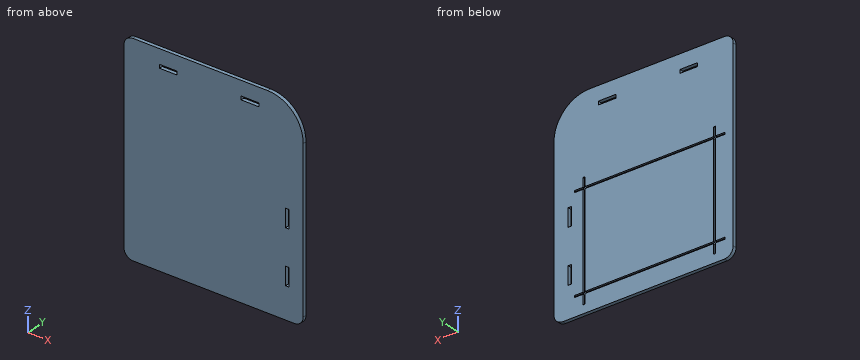
```python
from build123d import *

# Parameters (mm, degrees)
SKETCH1_W           = 20
SKETCH1_H           = 4
SKETCH1_W_2         = 4
SKETCH1_H_2         = 20
BOSS_EXTRUDE1_DEPTH = 4
SKETCH2_W           = 145
SKETCH2_H           = 105
CUT_EXTRUDE1_DEPTH  = 2


with BuildPart() as part:
    # Sketch1 → Boss-Extrude1 (new body)
    with BuildSketch(Plane(origin=(0, 0, 0), x_dir=(1, 0, 0), z_dir=(0, 1, 0))):
        with BuildLine():
            Line((-12.1, 127.1), (170, 127.1))
            ThreePointArc((170, 127.1), (177.071067812, 124.171067812), (180, 117.1))
            Line((180, 117.1), (180, -60))
            ThreePointArc((180, -60), (168.284271247, -88.284271247), (140, -100))
            Line((140, -100), (-12.1, -100))
            ThreePointArc((-12.1, -100), (-19.171067812, -97.071067812), (-22.1, -90))
            Line((-22.1, -90), (-22.1, 117.1))
            ThreePointArc((-22.1, 117.1), (-19.171067812, 124.171067812), (-12.1, 127.1))
        make_face()
        with Locations((27.9, -82)):
            Rectangle(SKETCH1_W, SKETCH1_H, mode=Mode.SUBTRACT)
        with Locations((120, -82)):
            Rectangle(SKETCH1_W, SKETCH1_H, mode=Mode.SUBTRACT)
        with Locations((162, 82.1)):
            Rectangle(SKETCH1_W_2, SKETCH1_H_2, mode=Mode.SUBTRACT)
        with Locations((162, 22.9)):
            Rectangle(SKETCH1_W_2, SKETCH1_H_2, mode=Mode.SUBTRACT)
    extrude(amount=BOSS_EXTRUDE1_DEPTH)

    # Sketch2 → Cut-Extrude1 (cut)
    with BuildSketch(Plane(origin=(0, 4, 0), x_dir=(1, 0, 0), z_dir=(0, 1, 0))):
        Polygon((-12.9, 0), (-2.1, 0), (-2.1, 105), (-12.9, 105), (-12.9, 107.1), (-2.1, 107.1), (-2.1, 117.9), (0, 117.9), (0, 107.1), (145, 107.1), (145, 117.9), (147.1, 117.9), (147.1, 107.1), (157.1, 107.1), (157.1, 105), (147.1, 105), (147.1, 0), (157.1, 0), (157.1, -2.1), (147.1, -2.1), (147.1, -12.1), (145, -12.1), (145, -2.1), (0, -2.1), (0, -12.1), (-2.1, -12.1), (-2.1, -2.1), (-12.9, -2.1), align=None)
        with Locations((72.5, 52.5)):
            Rectangle(SKETCH2_W, SKETCH2_H, mode=Mode.SUBTRACT)
    extrude(amount=-CUT_EXTRUDE1_DEPTH, mode=Mode.SUBTRACT)


solid = part.part
```
Design review of the part built by this model. Coordinates are the model's own, in mm. Round coordinates to 2 decimals unless told otherwise and drop trailing zeros. Order: outer loops, then holes, each group sorted by start corner. A loop starts at its lowest first (then second) coordinate and runs counter-clockwise, first axis right, second up. Notation, with made-up numbers: (0, -25) - (25, -25) arc R22 ccw to (25, 13) - close; hole circle Ø5 at (86.25, 81). An arc over 180 degrees is marked (long way). Return JSON: item names as keys, results as strings.
Q1. Wall thickness on L1, parallel to Z at x = 62, y = 2.05; L2, parallel to X at y = 2.1, z = 9.5; L3, parallel to Z at x = 117, y = 3.15: over which ranges is each line inside the solid? List them lowest first. Write a range as [from, to].
Computed values:
{"L1": "z = [-127.1, -107.1], [-105, 0], [2.1, 100]", "L2": "x = [-22.1, -2.1], [0, 145], [147.1, 180]", "L3": "z = [-127.1, -107.1], [-105, 0], [2.1, 80], [84, 100]"}
Q2. Consider section A-A on z = -80. Write out the cut boundary in (x, y), plus the area to 3 significant figures.
Computed values:
{"outline": "(-22.1, 0) - (160, 0) - (160, 4) - (147.1, 4) - (147.1, 2) - (145, 2) - (145, 4) - (0, 4) - (0, 2) - (-2.1, 2) - (-2.1, 4) - (-22.1, 4) - close; (164, 0) - (180, 0) - (180, 4) - (164, 4) - close", "area": "784 mm2"}
Q3. Consider section C-C on y = 1. Write out the cut boundary in (x, z), plus the area to 3 significant figures.
Computed values:
{"outline": "(-22.1, -117.1) arc R10 ccw to (-12.1, -127.1) - (170, -127.1) arc R10 ccw to (180, -117.1) - (180, 60) arc R40 ccw to (140, 100) - (-12.1, 100) arc R10 ccw to (-22.1, 90) - close; hole (17.9, 80) - (37.9, 80) - (37.9, 84) - (17.9, 84) - close; hole (110, 80) - (130, 80) - (130, 84) - (110, 84) - close; hole (160, -92.1) - (164, -92.1) - (164, -72.1) - (160, -72.1) - close; hole (160, -32.9) - (164, -32.9) - (164, -12.9) - (160, -12.9) - close", "area": "45,200 mm2"}
Q4. For pin 1 Ø2 at (y, z) = (1.5, 82.5) entering from +X, flat-tipped, find the tip position at first contact; note if it passes through.
Computed values:
{"pin 1": "stops at x = 173.73"}
Q5. Consider section D-D on z = 77. Write out the cut boundary in (x, y).
Computed values:
{"outline": "(-22.1, 0) - (176.21, 0) - (176.21, 4) - (-22.1, 4) - close"}
Q6. Consider section B-B on x = 27.5. Write out the cut boundary in (y, z), plus the area to 3 significant figures.
Computed values:
{"outline": "(0, -127.1) - (4, -127.1) - (4, -107.1) - (2, -107.1) - (2, -105) - (4, -105) - (4, 0) - (2, 0) - (2, 2.1) - (4, 2.1) - (4, 80) - (0, 80) - close; (0, 84) - (4, 84) - (4, 100) - (0, 100) - close", "area": "884 mm2"}
